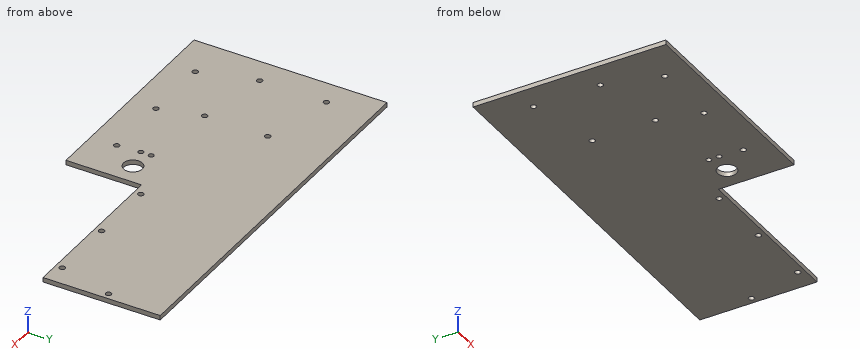
```python
from build123d import *

# Parameters (mm, degrees)
BOSS_EXTRUDE1_DEPTH   = 3.1
F_6_CLEARANCE_HOLE1_D = 3.7973
F_6_CLEARANCE_HOLE2_D = 3.7973
SKETCH8_R             = 6.35
SKETCH8_R_2           = 1.75
CUT_EXTRUDE1_DEPTH    = 4.1


with BuildPart() as part:
    # Sketch1 → Boss-Extrude1 (new body)
    with BuildSketch(Plane.XY):
        Polygon((130, -14), (16.9, -14), (16.9, -65), (-130, -65), (-130, 65), (130, 65), align=None)
    extrude(amount=BOSS_EXTRUDE1_DEPTH)

    # #6 Clearance Hole1 (through all)
    with Locations(Plane.XY.offset(3.1)):
        with Locations((25.5, -9.5), (70.5, -9.5), (115.5, -9.5), (-11.54975, -47.5), (-56.54975, -47.5), (-101.54975, -47.5), (125.5, 27.5), (-64.244394137, -19.232770082), (-64.244394137, 23.267229918)):
            Hole(F_6_CLEARANCE_HOLE1_D / 2)

    # #6 Clearance Hole2 (through all)
    with Locations(Plane.XY.offset(3.1)):
        with Locations((-112.4995, 34.5024), (-112.4995, -10.4976)):
            Hole(F_6_CLEARANCE_HOLE2_D / 2)

    # Sketch8 → Cut-Extrude1 (cut, through all)
    with BuildSketch(Plane(origin=(0, 0, 0), x_dir=(-1, 0, 0), z_dir=(0, 0, -1))):
        with Locations((-2.31737005, -28.419585766)):
            Circle(SKETCH8_R)
        with Locations((12.68262995, -24.919585766)):
            Circle(SKETCH8_R_2)
        with Locations((12.68262995, -31.919585766)):
            Circle(SKETCH8_R_2)
    extrude(amount=-CUT_EXTRUDE1_DEPTH, mode=Mode.SUBTRACT)


solid = part.part
```
The model under review builds one solid part; all positions refer to its coordinate system, in mm. Round coordinates to 2 decimals unless told otherwise and drop trailing zeros. Order: outer loops, then holes, each group sorted by start corner. A loop starts at its lowest first (then second) coordinate and runs counter-clockwise, first axis right, second up. Notation, with made-up numbers: (56, 15) - (65, 15) arc R5 ccw to (65, 24) - close; hole circle Ø4 at (64.5, 31). An arc over 180 degrees is marked (long way). Answer in a Markdown table with one row per item.
(1) Clearance check with flat-ended pins moving along their axes: P1, Ø2.5, axis at x = -101.55, y = -47.5, coming from the -Z side; P2, Ø6, axis at x = 125.5, y = 27.5, coming from the -Z side; P3, Ø0.9, axis at y = -44.5, z = 1.5, coming from the +X side; P4, Ø1.6, axis at x = 56, z = 1.5, coming from the -Y side. State where each tip first meets the part, or that it passes through.
Result set:
| item | result |
|---|---|
| P1 | passes through |
| P2 | stops at z = 0 |
| P3 | stops at x = 16.9 |
| P4 | stops at y = -14 |
(2) Take a section at C-C on x = 31.5. Write out the cut boundary in (y, z).
Result set:
| item | result |
|---|---|
| outline | (-14, 0) - (65, 0) - (65, 3.1) - (-14, 3.1) - close |
(3) For line 1 (Y direction, x = 125.5, z = 2.15); line 2 (X direction, y = -9, z = 1.6); line 3 (Y direction, x = 70.5, z = 0.75), list the stretches that pass through material, from the lowest coordinate up. Write a range as from..to.
Result set:
| item | result |
|---|---|
| line 1 | y = -14..25.6, 29.4..65 |
| line 2 | x = -130..-113.67, -111.33..23.67, 27.33..68.67, 72.33..113.67, 117.33..130 |
| line 3 | y = -14..-11.4, -7.6..65 |
(4) Take a section at A-A on z = 0.7. Count the separate pieces of the cut face and the enclosed holes in it, plus the area to 3 significant figures.
Result set:
| item | result |
|---|---|
| separate pieces | 1 |
| enclosed holes | 14 |
| area | 27,800 mm2 |
(5) Take a section at B-B on y = -43. Write out the cut boundary in (x, z), plus the area to 3 significant figures.
Result set:
| item | result |
|---|---|
| outline | (-130, 0) - (16.9, 0) - (16.9, 3.1) - (-130, 3.1) - close |
| area | 455 mm2 |
